CAD build for the part. Positions are in the model's coordinates, mm. Face numbers are marked on the shaded views. A direction names the side the tool comes from. Coordinates: 2 decimals unless noted, no trailing zeros. Loops run counter-clockwise (first coordinate to the right, second up) from the corner with the lowest first, then second, coordinate; pieces in that order, holes last. Notation, with made-up numbers: (74.5, 4.5) -> (125.5, 4.5) arc R20 ccw to (125.5, 38.5) -> close; hole circle Ø5 at (36.25, 29.25). An arc over 180 degrees is marked (long way). Write each question's results on one line, items separated by ' | '.
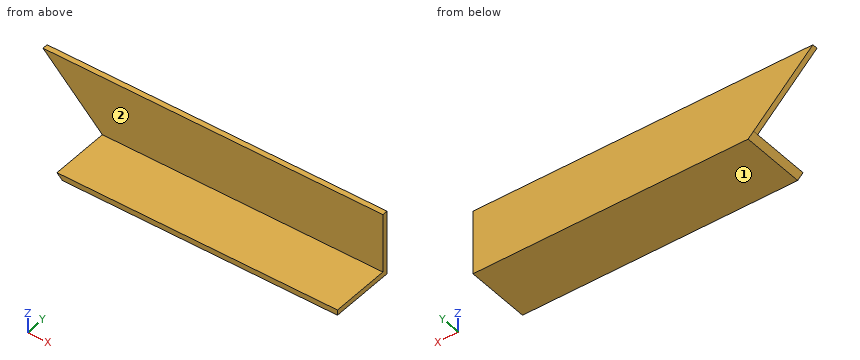
```python
from build123d import *

# Parameters (mm, degrees)
F1_DEPTH = 6.35
F0_W     = 330.2
F0_H     = 6.35
F2_DEPTH = 76.2
F3_SIZE  = 6.34999


# Not quite as in the source:
# - a fillet or chamfer is up to 0.001 mm smaller than in the source, because OpenCascade refuses the exact size


with BuildPart() as f1:
    # F0 (on Front) → F1 (new body)
    with BuildSketch(Plane.XZ):
        Polygon((-339.7388204469, 69.3321084814), (-269.8888204469, -0.5178915186), (60.3111795531, -0.5178915186), (60.3111795531, 69.3321084814), align=None)
    extrude(amount=F1_DEPTH)

    # F0 (on Front) → F2 (join)
    with BuildSketch(Plane.XZ):
        with Locations((-104.7888204469, -3.6928915186)):
            Rectangle(F0_W, F0_H)
    extrude(amount=F2_DEPTH)

    # F3 (size 6.35 in the source; OpenCascade refuses exactly that, so slightly less here)
    f3_edges = [f1.edges().sort_by_distance(p)[0] for p in [
        (-269.88882, -38.1, -6.867892),
    ]]
    chamfer(f3_edges, length=F3_SIZE)


solid = f1.part
```
Q1. Wall check: L1, parallel to Y at x = -70, z = 41; L2, parallel to Z at x = -212.5, y = -54.5; L3, parallel to Z at x = -304, y = -4. Give the ranges that are in metal, low to high. Write a range as from..to.
Results are:
L1: -6.35..0 | L2: -6.87..-0.52 | L3: 33.59..69.33
Q2. Cut at C-C on z = 32. Write the cut outline in (x, y).
Results are:
outline: (-302.41, -6.35) -> (60.31, -6.35) -> (60.31, 0) -> (-302.41, 0) -> close
Q3. Drop flat-ended pins along their axis: pin 1 (5 mm diameter, centred on x = 7.5, z = 30.5, fed in from -Y); pin 2 (10 mm diameter, centred on x = -32, y = -67, fed in from +Z). Give the stop position or say it passes through.
Results are:
pin 1: y = -6.35 | pin 2: z = -0.52
Q4. Cut at A-A on x = -241. Write the cut outline in (y, z).
Results are:
outline: (-76.2, -6.87) -> (0, -6.87) -> (0, 69.33) -> (-6.35, 69.33) -> (-6.35, -0.52) -> (-76.2, -0.52) -> close
Q5. Which spindle directions (+Z, -Z, +X, -X, +Y, -Y) get a long thin tool onto all of the face, cutting with end or side? Do the marked faces 1 and 2. Say none if no direction does.
Results are:
face 1: -Z, +X, -X, +Y, -Y | face 2: +Z, +X, -X, -Y
Q6. Cut at D-D on z = 51. Write the cut outline in (x, y).
Results are:
outline: (-321.41, -6.35) -> (60.31, -6.35) -> (60.31, 0) -> (-321.41, 0) -> close
